Here's the drawing with two shaded views (mm, measured from the low corner). I have some questions. Round coordinates to 2 decimals unless told otherwise and drop trailing zeros. Write each loop counter-clockwise with the first axis right and the second up, starting at its lowest first coordinate (ties: lowest second). Pieces come first, ordered by that corner, then holes. Notation, with made-up numbers: M 51.5,-38.75 L 100.5,-38.75 A27 ccw 100.5,-5.75 Z; hole C 4.25,62 d2. An arc over 180 degrees is marked long. Write item = value, one per line. Start each with the question number.
(1) I need wall thicknesses on line 1 along Y through (x, z) = (19.7, 7.75); line 2 along Y through (x, z) = (21.5, 28.75); line 3 along X through (y, z) = (28, 26.25). Which ranges of each line are inside material? Lowest first, please.
(2) I want a section at C-C (y = 36.5). List the corners of the cut face in (x, z) for me.
(3) Will these pins go through, and if not, where does the flat tip stop? pin 1 Ø3.5 at (x, y) = (35.879, 19.7) entering from +Z; pin 2 Ø1 at (x, z) = (26, 23) entering from +Y; pin 3 Ø4 at (y, z) = (27.5, 26.5) entering from +X; pin 4 Ø8 at (x, z) = (29, 19) entering from -Y.
(4) I want a section at D-D (x = 24). List the corners of the cut face in (y, z) for me.
(5) If we mould it in two halves opening along X, with no side actions, what happens to the marked faces 1, 2 and 3? For each: released by +X, released by -X, zero draft, split by the parting line, or undercut.
(6) I want a section at A-A (x = 19.7). List the corners of the cut face in (y, z) for me, and give its area (3 significant figures).
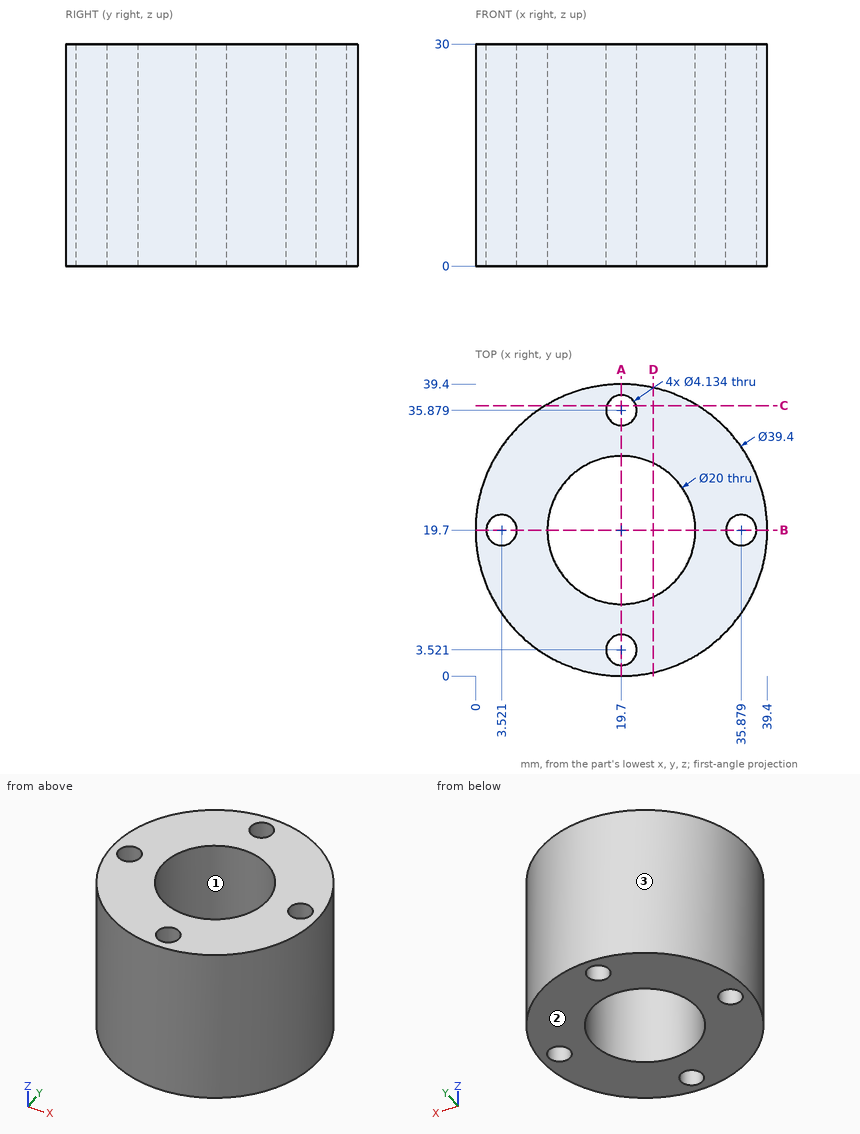
Returned:
q1.line_1 = 0 to 1.45, 5.59 to 9.7, 29.7 to 33.81, 37.95 to 39.4
q1.line_2 = 0.08 to 2.5, 4.54 to 9.86, 29.54 to 34.86, 36.9 to 39.32
q1.line_3 = 1.83 to 14.12, 25.28 to 37.57
q2.outline = M 9.41,0 L 17.73,0 L 17.73,30 L 9.41,30 Z; M 21.67,0 L 29.99,0 L 29.99,30 L 21.67,30 Z
q3.pin_1 = through
q3.pin_2 = 38.53
q3.pin_3 = 38.53
q3.pin_4 = 0.73
q4.outline = M 0.48,0 L 10.67,0 L 10.67,30 L 0.48,30 Z; M 28.73,0 L 38.92,0 L 38.92,30 L 28.73,30 Z
q5.face_1 = undercut
q5.face_2 = zero draft
q5.face_3 = split by the parting line
q6.outline = M 0,0 L 1.45,0 L 1.45,30 L 0,30 Z; M 5.59,0 L 9.7,0 L 9.7,30 L 5.59,30 Z; M 29.7,0 L 33.81,0 L 33.81,30 L 29.7,30 Z; M 37.95,0 L 39.4,0 L 39.4,30 L 37.95,30 Z
q6.area = 334 mm²
